from build123d import *

# Parameters (mm, degrees)
SKETCH1_W           = 170
SKETCH1_H           = 110
BOSS_EXTRUDE1_DEPTH = 2
SKETCH2_W           = 166
SKETCH2_H           = 106
SKETCH2_W_2         = 160
SKETCH2_H_2         = 100
BOSS_EXTRUDE3_DEPTH = 5


with BuildPart() as part:
    # Sketch1 → Boss-Extrude1 (new body)
    with BuildSketch(Plane.XY):
        Rectangle(SKETCH1_W, SKETCH1_H)
    extrude(amount=BOSS_EXTRUDE1_DEPTH)

    # Sketch2 → Boss-Extrude3 (add)
    with BuildSketch(Plane.XY.offset(2)):
        Rectangle(SKETCH2_W, SKETCH2_H)
        Rectangle(SKETCH2_W_2, SKETCH2_H_2, mode=Mode.SUBTRACT)
    extrude(amount=-BOSS_EXTRUDE3_DEPTH)


solid = part.part
Geometry: final body of the model. Coordinates: model frame, mm. Give positions to 0.01 mm unless a question says otherwise; leave off trailing zeros. Write each loop counter-clockwise with the first axis right and the second up, starting at its lowest first coordinate (ties: lowest second). Pieces come first, ordered by that corner, then holes. Notation, with made-up numbers: M 33.5,-4 L 48.5,-4 A19 ccw 48.5,28 Z; hole C -35.5,-21 d10. An arc over 180 degrees is marked long. Answer in a Markdown table with one row per item. Add a question column.
(1) First-contact query: pin 1 (0.9 mm diameter, centred on y = -15, z = -1, fed in from +X); pin 2 (2.5 mm diameter, centred on x = 4, z = -2, fed in from +Y); pin 3 (2.5 mm diameter, centred on x = 6, z = -2, fed in from -Y). Flat tips, straight axial feed; report the tip coordinate or a pass-through.
(2) Section A-A on z = -2.15. Return loops of the section in (x, y), and give its area (3 significant figures).
(3) Section B-B on x = 13.5. Return loops of the section in (y, z).
(4) Ray query, line 1 (X direction, y = 18, z = -0.8); line 2 (Y direction, x = 42, z = -1.25); line 3 (Z direction, x = 38.5, y = 42.5). Return the intervals inside material, ascending.
(5) Section C-C on y = 30. Return loops of the section in (x, z).
(6) Mould query, pull axis Y, two halves, no side actions, for faces 1 (the flat face through (-1, 1, 0)), 2 (the flat face through (-1, 1, 2)). Classes: +Y half, -Y half, draft (parallel to the pull), parting line (faces both ways), or undercut.
Result set:
| question | item | result |
|---|---|---|
| 1 | pin 1 | stops at x = 83 |
| 1 | pin 2 | stops at y = 53 |
| 1 | pin 3 | stops at y = -53 |
| 2 | outline | M -83,-53 L 83,-53 L 83,53 L -83,53 Z; hole M -80,-50 L 80,-50 L 80,50 L -80,50 Z |
| 2 | area | 1,600 mm^2 |
| 3 | outline | M -55,0 L -53,0 L -53,-3 L -50,-3 L -50,0 L 50,0 L 50,-3 L 53,-3 L 53,0 L 55,0 L 55,2 L -55,2 Z |
| 4 | line 1 | x = -83 to -80, 80 to 83 |
| 4 | line 2 | y = -53 to -50, 50 to 53 |
| 4 | line 3 | z = 0 to 2 |
| 5 | outline | M -85,0 L -83,0 L -83,-3 L -80,-3 L -80,0 L 80,0 L 80,-3 L 83,-3 L 83,0 L 85,0 L 85,2 L -85,2 Z |
| 6 | face 1 | undercut |
| 6 | face 2 | draft |
